Work out the finished part from the listing and answer in its coordinate system (mm). Coordinates: 2 decimals unless noted, no trailing zeros. Order: outer loops, then holes, each group sorted by start corner. A loop starts at its lowest first (then second) coordinate and runs counter-clockwise, first axis right, second up. Notation, with made-up numbers: (-13.75, -33.5) -> (-4.75, -33.5) arc R36 ccw to (-4.75, 0.5) -> close; hole circle Ø8 at (-15.5, 70). An arc over 180 degrees is marked (long way). Use one line per item in the form item = value.
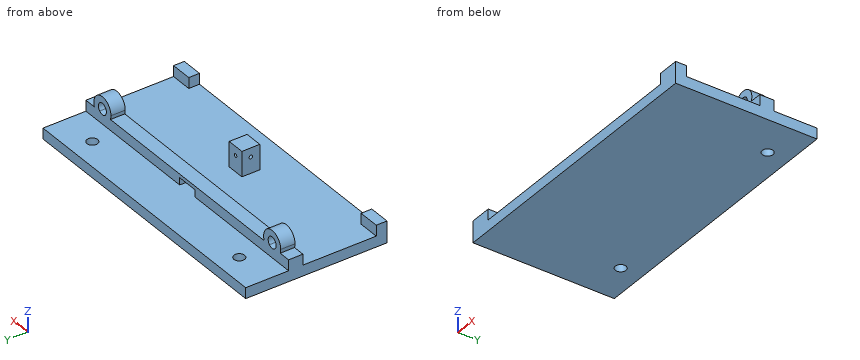
from build123d import *

# Parameters (mm, degrees)
F0_W      = 80
F0_H      = 27.5
F1_DEPTH  = 3
F2_W      = 80
F2_H      = 4
F2_W_2    = 6
F2_H_2    = 3
F3_DEPTH  = 3
F2_W_3    = 5
F2_H_3    = 5
F4_DEPTH  = 7
F5_R      = 0.5
F6_DEPTH  = 5
F7_W      = 6
F7_H      = 2
F8_DEPTH  = 4
F10_DEPTH = 4
F11_DEPTH = 4
F12_DEPTH = 4
F13_DEPTH = 4
F15_DEPTH = 12
F16_R     = 1.5
F17_DEPTH = 3
F18_R     = 0.5
F19_DEPTH = 42.501


with BuildPart() as f1:
    # F0 (on Top) → F1 (new body)
    with BuildSketch(Plane.XY):
        Rectangle(F0_W, F0_H)
    extrude(amount=F1_DEPTH)

    # F2 (on face) → F3 (join)
    with BuildSketch(Plane.XY.offset(3)):
        with Locations((0, 11.75)):
            Rectangle(F2_W, F2_H)
        with Locations((-37, -12.25)):
            Rectangle(F2_W_2, F2_H_2)
        with Locations((37, -12.25)):
            Rectangle(F2_W_2, F2_H_2)
    extrude(amount=F3_DEPTH)

    # F2 (on face) → F4 (join)
    with BuildSketch(Plane.XY.offset(3)):
        with Locations((0, -2.25)):
            Rectangle(F2_W_3, F2_H_3)
    extrude(amount=F4_DEPTH)

    # F5 (on face) → F6 (cut)
    with BuildSketch(Plane.XZ.offset(4.75)):
        with Locations((0, 7.5)):
            Circle(F5_R)
    extrude(amount=-F6_DEPTH, mode=Mode.SUBTRACT)

    # F7 (on face) → F8 (cut, through all)
    with BuildSketch(Plane(origin=(0, 13.75, 0), x_dir=(-1, 0, 0), z_dir=(0, 1, 0))):
        with Locations((0, 4)):
            Rectangle(F7_W, F7_H)
    extrude(amount=-F8_DEPTH, mode=Mode.SUBTRACT)

    # F9 (on face) → F10 (join)
    with BuildSketch(Plane(origin=(0, 13.75, 0), x_dir=(-1, 0, 0), z_dir=(0, 1, 0))):
        with BuildLine():
            ThreePointArc((-30.3269691146, 6), (-30.1758757365, 6.5661996225), (-30.125, 7.15))
            ThreePointArc((-30.125, 7.15), (-34.0838003775, 10.4741242635), (-36.6730308854, 6))
            Line((-36.6730308854, 6), (-34.5761621625, 6))
            ThreePointArc((-34.5761621625, 6), (-34.1267653445, 8.5949187531), (-31.925, 7.15))
            ThreePointArc((-31.925, 7.15), (-32.0550812469, 6.5232346555), (-32.4238378375, 6))
            Line((-32.4238378375, 6), (-30.3269691146, 6))
        make_face()
        with BuildLine():
            Line((-34.5761621625, 6), (-36.6730308854, 6))
            ThreePointArc((-36.6730308854, 6), (-33.5, 3.775), (-30.3269691146, 6))
            Line((-30.3269691146, 6), (-32.4238378375, 6))
            ThreePointArc((-32.4238378375, 6), (-33.5, 5.575), (-34.5761621625, 6))
        make_face()
        with BuildLine():
            Line((-32.4238378375, 6), (-34.5761621625, 6))
            ThreePointArc((-34.5761621625, 6), (-33.5, 5.575), (-32.4238378375, 6))
        make_face()
        with BuildLine():
            ThreePointArc((-31.925, 7.15), (-34.1267653445, 8.5949187531), (-34.5761621625, 6))
            Line((-34.5761621625, 6), (-32.4238378375, 6))
            ThreePointArc((-32.4238378375, 6), (-32.0550812469, 6.5232346555), (-31.925, 7.15))
        make_face()
    extrude(amount=-F10_DEPTH)

    # F9 (on face) → F11 (cut, through all)
    with BuildSketch(Plane(origin=(0, 13.75, 0), x_dir=(-1, 0, 0), z_dir=(0, 1, 0))):
        with BuildLine():
            Line((-32.4238378375, 6), (-34.5761621625, 6))
            ThreePointArc((-34.5761621625, 6), (-33.5, 5.575), (-32.4238378375, 6))
        make_face()
        with BuildLine():
            ThreePointArc((-31.925, 7.15), (-34.1267653445, 8.5949187531), (-34.5761621625, 6))
            Line((-34.5761621625, 6), (-32.4238378375, 6))
            ThreePointArc((-32.4238378375, 6), (-32.0550812469, 6.5232346555), (-31.925, 7.15))
        make_face()
    extrude(amount=-F11_DEPTH, mode=Mode.SUBTRACT)

    # F9 (on face) → F12 (join)
    with BuildSketch(Plane(origin=(0, 13.75, 0), x_dir=(-1, 0, 0), z_dir=(0, 1, 0))):
        with BuildLine():
            ThreePointArc((36.875, 7.15), (32.9161996225, 10.4741242635), (30.3269691146, 6))
            Line((30.3269691146, 6), (32.4238378375, 6))
            ThreePointArc((32.4238378375, 6), (32.8732346555, 8.5949187531), (35.075, 7.15))
            ThreePointArc((35.075, 7.15), (34.9449187531, 6.5232346555), (34.5761621625, 6))
            Line((34.5761621625, 6), (36.6730308854, 6))
            ThreePointArc((36.6730308854, 6), (36.8241242635, 6.5661996225), (36.875, 7.15))
        make_face()
        with BuildLine():
            ThreePointArc((35.075, 7.15), (32.8732346555, 8.5949187531), (32.4238378375, 6))
            Line((32.4238378375, 6), (34.5761621625, 6))
            ThreePointArc((34.5761621625, 6), (34.9449187531, 6.5232346555), (35.075, 7.15))
        make_face()
        with BuildLine():
            Line((34.5761621625, 6), (32.4238378375, 6))
            ThreePointArc((32.4238378375, 6), (33.5, 5.575), (34.5761621625, 6))
        make_face()
        with BuildLine():
            Line((32.4238378375, 6), (30.3269691146, 6))
            ThreePointArc((30.3269691146, 6), (33.5, 3.775), (36.6730308854, 6))
            Line((36.6730308854, 6), (34.5761621625, 6))
            ThreePointArc((34.5761621625, 6), (33.5, 5.575), (32.4238378375, 6))
        make_face()
    extrude(amount=-F12_DEPTH)

    # F9 (on face) → F13 (cut, through all)
    with BuildSketch(Plane(origin=(0, 13.75, 0), x_dir=(-1, 0, 0), z_dir=(0, 1, 0))):
        with BuildLine():
            ThreePointArc((35.075, 7.15), (32.8732346555, 8.5949187531), (32.4238378375, 6))
            Line((32.4238378375, 6), (34.5761621625, 6))
            ThreePointArc((34.5761621625, 6), (34.9449187531, 6.5232346555), (35.075, 7.15))
        make_face()
        with BuildLine():
            Line((34.5761621625, 6), (32.4238378375, 6))
            ThreePointArc((32.4238378375, 6), (33.5, 5.575), (34.5761621625, 6))
        make_face()
    extrude(amount=-F13_DEPTH, mode=Mode.SUBTRACT)

    # F14 (on face) → F15 (join)
    with BuildSketch(Plane(origin=(0, 13.75, 0), x_dir=(-1, 0, 0), z_dir=(0, 1, 0))):
        Polygon((-40, 3), (-40, 0), (40, 0), (40, 3), (3, 3), (-3, 3), align=None)
    extrude(amount=F15_DEPTH)

    # F16 (on face) → F17 (cut, through all)
    with BuildSketch(Plane.XY.offset(3)):
        with Locations((29, 19.75)):
            Circle(F16_R)
        with Locations((-29, 19.75)):
            Circle(F16_R)
    extrude(amount=-F17_DEPTH, mode=Mode.SUBTRACT)

    # F18 (on face) → F19 (cut, through all)
    with BuildSketch(Plane(origin=(-2.5, 0, 0), x_dir=(0, -1, 0), z_dir=(-1, 0, 0))):
        with Locations((2.25, 7.5)):
            Circle(F18_R)
    extrude(amount=-F19_DEPTH, mode=Mode.SUBTRACT)


solid = f1.part
(1) Straight lines are drawn through the part: line 1 along Z through (x, y) = (2.05, -2.25); line 2 along X through (y, z) = (-0.4, 7.5); line 3 along Y through (x, z) = (29, 2.45). For each, find the intervals that lie inside material, in ascending order.
Data:
line_1 = 0 to 7, 8 to 10
line_2 = -2.5 to -0.5, 0.5 to 2.5
line_3 = -13.75 to 18.25, 21.25 to 25.75
(2) Section B-B on y = -4 is taken. Write down the section's boundary in (x, z), plus the area to 3 significant figures.
Data:
outline = (-40, 0) -> (40, 0) -> (40, 3) -> (2.5, 3) -> (2.5, 10) -> (-2.5, 10) -> (-2.5, 3) -> (-40, 3) -> close; hole circle Ø1 at (0, 7.5)
area = 274 mm²
(3) Each of these flat-tipped pins is pushed along its axis until it touches: P1, Ø10, axis at x = 25, y = -3, coming from the +Z side; P2, Ø3.5, axis at x = -36.5, y = -12.5, coming from the +Z side; P3, Ø4, axis at y = -3.5, z = 8, coming from the -X side; P4, Ø2.5, axis at x = -29, y = 19.75, coming from the -Z side. Where does it stop, or does it pass through?
Data:
P1 = 3
P2 = 6
P3 = -2.5
P4 = through
(4) Section A-A on y = 19.75 is taken. Write down the section's boundary in (x, z), plus the area to 3 significant figures.
Data:
outline = (-40, 0) -> (-30.5, 0) -> (-30.5, 3) -> (-40, 3) -> close; (-27.5, 0) -> (27.5, 0) -> (27.5, 3) -> (-27.5, 3) -> close; (30.5, 0) -> (40, 0) -> (40, 3) -> (30.5, 3) -> close
area = 222 mm²
(5) Section C-C on x = 29 is taken. Write down the section's boundary in (y, z), plus the area to 4 significant figures.
Data:
outline = (-13.75, 0) -> (18.25, 0) -> (18.25, 3) -> (13.75, 3) -> (13.75, 6) -> (9.75, 6) -> (9.75, 3) -> (-13.75, 3) -> close; (21.25, 0) -> (25.75, 0) -> (25.75, 3) -> (21.25, 3) -> close
area = 121.5 mm²
(6) Section D-D on y = 10.5 is taken. Write down the section's boundary in (x, z) (3 decimals).
Data:
outline = (-40, 0) -> (40, 0) -> (40, 6) -> (36.673, 6) arc R3.375 ccw (long way) to (30.327, 6) -> (-30.327, 6) arc R3.375 ccw (long way) to (-36.673, 6) -> (-40, 6) -> close; hole circle Ø3.15 at (-33.5, 7.15); hole (-3, 3) -> (3, 3) -> (3, 5) -> (-3, 5) -> close; hole circle Ø3.15 at (33.5, 7.15)
